from build123d import *

# Parameters (mm, degrees)
SKETCH1_W           = 54
SKETCH1_H           = 26.5
BOSS_EXTRUDE1_DEPTH = 5
SKETCH2_W           = 6.5
SKETCH2_H           = 10
BOSS_EXTRUDE2_DEPTH = 19.5
SKETCH3_R           = 2.06
CUT_EXTRUDE1_DEPTH  = 19
SKETCH4_R           = 2.06
BOSS_EXTRUDE3_DEPTH = 10
FILLET1_R           = 1
FILLET2_R           = 2
SKETCH5_W           = 54
SKETCH5_H           = 5
BOSS_EXTRUDE4_DEPTH = 13
SKETCH6_R           = 2.25
CUT_EXTRUDE2_DEPTH  = 15
FILLET3_R           = 2
SKETCH7_R           = 4
SKETCH7_R_2         = 2.25
BOSS_EXTRUDE5_DEPTH = 5


with BuildPart() as part:
    # Sketch1 → Boss-Extrude1 (new body)
    with BuildSketch(Plane.XY):
        Rectangle(SKETCH1_W, SKETCH1_H)
    extrude(amount=BOSS_EXTRUDE1_DEPTH)

    # Sketch2 → Boss-Extrude2 (add)
    with BuildSketch(Plane(origin=(0, 0, 0), x_dir=(-1, 0, 0), z_dir=(0, 0, -1))):
        with Locations((-23.75, -8.25)):
            Rectangle(SKETCH2_W, SKETCH2_H)
        with Locations((23.75, -8.25)):
            Rectangle(SKETCH2_W, SKETCH2_H)
    extrude(amount=BOSS_EXTRUDE2_DEPTH)

    # Sketch3 → Cut-Extrude1 (cut)
    with BuildSketch(Plane.XZ.offset(13.25)):
        with Locations((23.9, -15.6)):
            Circle(SKETCH3_R)
        with Locations((-23.9, -5.4)):
            Circle(SKETCH3_R)
        with Locations((23.9, -5.4)):
            Circle(SKETCH3_R)
        with Locations((-23.9, -15.6)):
            Circle(SKETCH3_R)
    extrude(amount=-CUT_EXTRUDE1_DEPTH, mode=Mode.SUBTRACT)

    # Sketch4 → Boss-Extrude3 (add)
    with BuildSketch(Plane.XZ.offset(13.25)):
        with BuildLine():
            Line((20.5, -17.926886332), (20.5, -13.273113668))
            ThreePointArc((20.5, -13.273113668), (28.02, -15.6), (20.5, -17.926886332))
        make_face()
        with Locations((23.9, -15.6)):
            Circle(SKETCH4_R, mode=Mode.SUBTRACT)
        with BuildLine():
            Line((20.5, -7.726886332), (20.5, -3.073113668))
            ThreePointArc((20.5, -3.073113668), (28.02, -5.4), (20.5, -7.726886332))
        make_face()
        with Locations((23.9, -5.4)):
            Circle(SKETCH4_R, mode=Mode.SUBTRACT)
        with BuildLine():
            Line((-20.5, -7.726886332), (-20.5, -3.073113668))
            ThreePointArc((-20.5, -3.073113668), (-28.02, -5.4), (-20.5, -7.726886332))
        make_face()
        with Locations((-23.9, -5.4)):
            Circle(SKETCH4_R, mode=Mode.SUBTRACT)
        with BuildLine():
            Line((-20.5, -17.926886332), (-20.5, -13.273113668))
            ThreePointArc((-20.5, -13.273113668), (-28.02, -15.6), (-20.5, -17.926886332))
        make_face()
        with Locations((-23.9, -15.6)):
            Circle(SKETCH4_R, mode=Mode.SUBTRACT)
    extrude(amount=-BOSS_EXTRUDE3_DEPTH)

    # Fillet1
    fillet1_edges = [part.edges().sort_by_distance(p)[0] for p in [
        (20.5, -8.25, 0),
        (-20.5, -8.25, 0),
    ]]
    fillet(fillet1_edges, radius=FILLET1_R)

    # Fillet2
    fillet2_edges = [part.edges().sort_by_distance(p)[0] for p in [
        (23.75, -3.25, 0),
        (-23.75, -3.25, 0),
    ]]
    fillet(fillet2_edges, radius=FILLET2_R)

    # Sketch5 → Boss-Extrude4 (add)
    with BuildSketch(Plane.XZ.offset(13.25)):
        with Locations((0, 2.5)):
            Rectangle(SKETCH5_W, SKETCH5_H)
    extrude(amount=BOSS_EXTRUDE4_DEPTH)

    # Sketch6 → Cut-Extrude2 (cut)
    with BuildSketch(Plane(origin=(0, 0, 0), x_dir=(-1, 0, 0), z_dir=(0, 0, -1))):
        with Locations((22, -24.25)):
            Circle(SKETCH6_R)
        with Locations((-22, -24.25)):
            Circle(SKETCH6_R)
    extrude(amount=-CUT_EXTRUDE2_DEPTH, mode=Mode.SUBTRACT)

    # Fillet3
    fillet3_edges = [part.edges().sort_by_distance(p)[0] for p in [
        (23.25, -13.25, 0),
        (-23.25, -13.25, 0),
    ]]
    fillet(fillet3_edges, radius=FILLET3_R)

    # Sketch7 → Boss-Extrude5 (add)
    with BuildSketch(Plane(origin=(0, 0, 0), x_dir=(-1, 0, 0), z_dir=(0, 0, -1))):
        with Locations((22, -24.25)):
            Circle(SKETCH7_R)
        with Locations((22, -24.25)):
            Circle(SKETCH7_R_2, mode=Mode.SUBTRACT)
        with Locations((-22, -24.25)):
            Circle(SKETCH7_R)
        with Locations((-22, -24.25)):
            Circle(SKETCH7_R_2, mode=Mode.SUBTRACT)
    extrude(amount=-BOSS_EXTRUDE5_DEPTH)


solid = part.part
Geometry: final body of the model. Coordinates: model frame, mm. A direction names the side the tool comes from. Coordinates: 2 decimals unless noted, no trailing zeros. Order: outer loops, then holes, each group sorted by start corner. A loop starts at its lowest first (then second) coordinate and runs counter-clockwise, first axis right, second up.
(1) Section query B-B (z = -5.4). Return the cut outline in (x, y), plus the area to 3 significant figures.
(2) First-contact query: pin 1 (4 mm diameter, centred on x = 9, z = 3.5, fed in from -Y); pin 2 (0.9 mm diameter, centred on x = 25.5, y = -9.5, fed in from -Z); pin 3 (2.5 mm diameter, centred on x = 23.9, z = -15.6, fed in from +Y); pin 4 (2.5 mm diameter, centred on y = -7, z = -11.5, fed in from +X). Flat tips, straight axial feed; report the tip coordinate or a pass-through.
(3) Access query for faces 5 (the face through (-27, -6, 2)), 6 (the face through (24, -3.25, -11)), 7 (the face through (-22, -8, -19.5)), 8 (the face through (22.06, -28.25, 2.46)), 9 (the face through (24, -13.25, -11)). Directions: +Z, -Z, +X, -X, +Y, -Y. A direction counts if a zero-diameter tool reaches every point of the face in a straight line with its end or side. Return the directions, or none.
(4) Draft query along X for faces 1 (the face through (27, -8, -19)), 2 (the face through (-26, -8, -19.5)), 3 (the face through (-27, -8, -19)), 4 (the face through (-20.5, -8, -10)). Return one class per face: pulls with the +X half, pulls with the -X half, needs draft (parallel to the pull), parting line crosses it, or undercut.
(5) Section query C-C (y = -7). Return the cut outline in (x, z), plus the area to 3 significant figures.
(6) Section query D-D (y = -24.25). Return the cut outline in (x, z), plus the area to 3 significant figures.
(7) Section query A-A (z = -11). Return the cut outline in (x, y).
(8) Material intervals for probe 1 along Y at (x, z) = (-22, 2.7); probe 2 along X at (y, z) = (-24.25, 3.95); probe 3 along Z at (x, y) = (23.9, -7.75), sorted ascending.
Solution:
1. outline: (-28.02, -13.25) - (-25.96, -13.25) - (-25.96, -3.25) - (-28.02, -3.25) - close; (-21.84, -13.25) - (-20.5, -13.25) - (-20.5, -3.25) - (-21.84, -3.25) - close; (20.5, -13.25) - (21.84, -13.25) - (21.84, -3.25) - (20.5, -3.25) - close; (25.96, -13.25) - (28.02, -13.25) - (28.02, -3.25) - (25.96, -3.25) - close
1. area: 68.0 mm2
2. pin 1: stops at y = -26.25
2. pin 2: stops at z = -19.56
2. pin 3: passes through
2. pin 4: stops at x = 27
3. face 5: +Z, -X, +Y, -Y
3. face 6: -Z, +X, -X, +Y
3. face 7: -Z, +Y, -Y
3. face 8: +Z, -Z, -Y
3. face 9: -Z, +X, -X, -Y
4. face 1: pulls with the +X half
4. face 2: needs draft
4. face 3: pulls with the -X half
4. face 4: undercut
5. outline: (-27, -19.5) - (-25.23, -19.5) arc R4.12 ccw to (-22.57, -19.5) - (-20.5, -19.5) - (-20.5, -1) arc R1 cw to (-19.5, 0) - (19.5, 0) arc R1 cw to (20.5, -1) - (20.5, -19.5) - (22.57, -19.5) arc R4.12 ccw to (25.23, -19.5) - (27, -19.5) - (27, -18.31) arc R4.12 ccw to (27, -12.89) - (27, -8.11) arc R4.12 ccw to (27, -2.69) - (27, 5) - (-27, 5) - (-27, -2.69) arc R4.12 ccw to (-27, -8.11) - (-27, -12.89) arc R4.12 ccw to (-27, -18.31) - close; hole circle Ø4.12 at (-23.9, -15.6); hole circle Ø4.12 at (-23.9, -5.4); hole circle Ø4.12 at (23.9, -15.6); hole circle Ø4.12 at (23.9, -5.4)
5. area: 487 mm2
6. outline: (-27, 0) - (-24.25, 0) - (-24.25, 5) - (-27, 5) - close; (-19.75, 0) - (19.75, 0) - (19.75, 5) - (-19.75, 5) - close; (24.25, 0) - (27, 0) - (27, 5) - (24.25, 5) - close
6. area: 225 mm2
7. outline: (-27, -13.25) - (-20.5, -13.25) - (-20.5, -3.25) - (-27, -3.25) - close; (20.5, -13.25) - (27, -13.25) - (27, -3.25) - (20.5, -3.25) - close
8. probe 1: y = -28.25 to -26.5, -22 to 13.25
8. probe 2: x = -27 to -24.25, -19.75 to 19.75, 24.25 to 27
8. probe 3: z = -19.72 to -17.66, -13.54 to -7.46, -3.34 to 5
